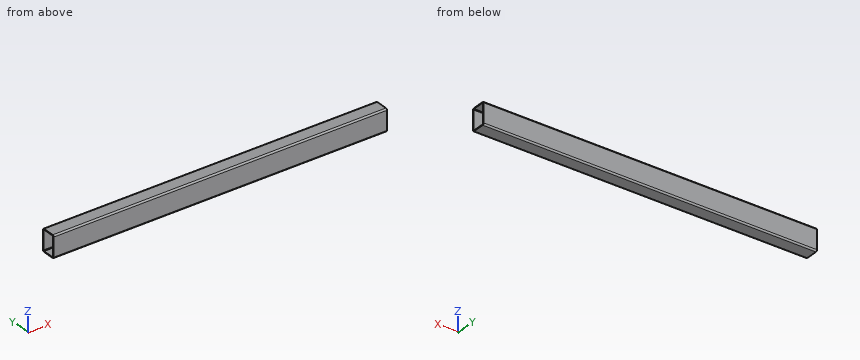
from build123d import *

# Parameters (mm, degrees)
F1_DEPTH = 2300


with BuildPart() as f1:
    # F0 (on Right) → F1 (new body)
    with BuildSketch(Plane.YZ):
        with BuildLine():
            ThreePointArc((50, 65), (47.071068, 72.071068), (40, 75))
            Line((40, 75), (-40, 75))
            ThreePointArc((-40, 75), (-47.071068, 72.071068), (-50, 65))
            Line((-50, 65), (-50, -65))
            ThreePointArc((-50, -65), (-47.071068, -72.071068), (-40, -75))
            Line((-40, -75), (40, -75))
            ThreePointArc((40, -75), (47.071068, -72.071068), (50, -65))
            Line((50, -65), (50, 65))
        make_face()
        with BuildLine():
            ThreePointArc((45, -65), (43.535534, -68.535534), (40, -70))
            Line((40, -70), (-40, -70))
            ThreePointArc((-40, -70), (-43.535534, -68.535534), (-45, -65))
            Line((-45, -65), (-45, 65))
            ThreePointArc((-45, 65), (-43.535534, 68.535534), (-40, 70))
            Line((-40, 70), (40, 70))
            ThreePointArc((40, 70), (43.535534, 68.535534), (45, 65))
            Line((45, 65), (45, -65))
        make_face(mode=Mode.SUBTRACT)
    extrude(amount=F1_DEPTH)


solid = f1.part
The listing builds one solid part. Answer for the finished solid, in the listing's coordinates (mm). Give positions to 0.01 mm unless a question says otherwise; leave off trailing zeros. Write each loop counter-clockwise with the first axis right and the second up, starting at its lowest first coordinate (ties: lowest second). Pieces come first, ordered by that corner, then holes. Notation, with made-up numbers: (-8.5, 37) - (7.5, 37) arc R22 cw to (7.5, 46) - close; hole circle Ø9 at (-34.75, 17.5). An arc over 180 degrees is marked (long way). Use a Markdown table: item, result.
1. Section C-C on x = 1113.5 is taken. Write down the section's boundary in (y, z), plus the area to 3 significant figures.
Values follow:
| item | result |
|---|---|
| outline | (-50, -65) arc R10 ccw to (-40, -75) - (40, -75) arc R10 ccw to (50, -65) - (50, 65) arc R10 ccw to (40, 75) - (-40, 75) arc R10 ccw to (-50, 65) - close; hole (-45, -65) arc R5 ccw to (-40, -70) - (40, -70) arc R5 ccw to (45, -65) - (45, 65) arc R5 ccw to (40, 70) - (-40, 70) arc R5 ccw to (-45, 65) - close |
| area | 2,340 mm² |
2. Section B-B on z = 18 is taken. Write down the section's boundary in (x, y).
Values follow:
| item | result |
|---|---|
| outline | (0, -50) - (2300, -50) - (2300, -45) - (0, -45) - close; (0, 45) - (2300, 45) - (2300, 50) - (0, 50) - close |
3. Section A-A on y = 20 is taken. Write down the section's boundary in (x, z).
Values follow:
| item | result |
|---|---|
| outline | (0, -75) - (2300, -75) - (2300, -70) - (0, -70) - close; (0, 70) - (2300, 70) - (2300, 75) - (0, 75) - close |
4. Find the intervals of material crossed by probe 1 along Z at (x, y) = (911, 21.5); probe 2 along Z at (x, y) = (2019, -42); probe 3 along Y at (x, z) = (606, -40), in increasing order. Write a range as from..to.
Values follow:
| item | result |
|---|---|
| probe 1 | z = -75..-70, 70..75 |
| probe 2 | z = -74.8..-69.58, 69.58..74.8 |
| probe 3 | y = -50..-45, 45..50 |
